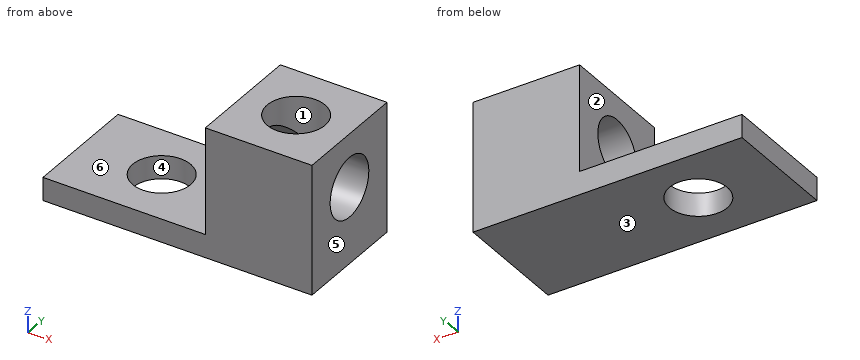
from build123d import *

# Parameters (mm, degrees)
EXTRUDE1_DEPTH      = 12.7
SKETCH2_R           = 3.27152
EXTRUDE2_DEPTH      = 27.071834918
EXTRUDE3_REACH      = 37.096
EXTRUDE3_END_RADIUS = 3.27152
SKETCH3_R           = 3.175
SKETCH4_R           = 3.175
EXTRUDE4_DEPTH      = 35.145763344


with BuildPart() as part:
    # Sketch1 → Extrude1 (new body)
    with BuildSketch(Plane(origin=(0, 0, 0), x_dir=(1, 0, 0), z_dir=(0, 1, 0))):
        Polygon((0, 0), (0, -14.224), (-11.684, -14.224), (-11.684, -2.54), (-29.464, -2.54), (-29.464, 0), align=None)
    extrude(amount=EXTRUDE1_DEPTH)

    # Sketch2 → Extrude2 (cut, through all)
    with BuildSketch(Plane.ZY.offset(11.684)):
        with Locations((8.382, 6.35)):
            Circle(SKETCH2_R)
    extrude(amount=-EXTRUDE2_DEPTH, mode=Mode.SUBTRACT)

    # Extrude3: up to this cylinder (the profile starts outside it)
    extrude3_end = Plane(origin=(-5.842, 6.35, 8.382), z_dir=(-1, 0, 0)) * Cylinder(EXTRUDE3_END_RADIUS, 81.73504, mode=Mode.PRIVATE)
    # Sketch3 → Extrude3 (cut, up to the surface)
    with BuildSketch(Plane.XY.offset(14.224), mode=Mode.PRIVATE) as extrude3_sk1:
        with Locations((-5.842, 6.35)):
            Circle(SKETCH3_R)
    extrude3_tool1 = extrude(extrude3_sk1.sketch, amount=-EXTRUDE3_REACH, mode=Mode.PRIVATE) - extrude3_end
    add(extrude3_tool1.solids().sort_by_distance((-5.842, 6.35, 14.224))[0], mode=Mode.SUBTRACT)

    # Sketch4 → Extrude4 (cut, through all)
    with BuildSketch(Plane.XY.offset(2.54)):
        with Locations((-20.574, 6.35)):
            Circle(SKETCH4_R)
    extrude(amount=-EXTRUDE4_DEPTH, mode=Mode.SUBTRACT)


solid = part.part
CAD build for the part. Positions are in the model's coordinates, mm. Face numbers are marked on the shaded views. A direction names the side the tool comes from. Round coordinates to 2 decimals unless told otherwise and drop trailing zeros. Write each loop counter-clockwise with the first axis right and the second up, starting at its lowest first coordinate (ties: lowest second). Pieces come first, ordered by that corner, then holes. Notation, with made-up numbers: M 79.25,49 L 126.25,49 A18 cw 126.25,54 Z; hole C 86.5,-17.5 d3. An arc over 180 degrees is marked long. Use a Markdown table: item, result. Add a question column.
1. Flat gauge pins, fed straight in: P1, Ø4, axis at x = -24.5, y = 4, coming from the +Z side; P2, Ø3.5, axis at y = 3.5, z = 8, coming from the -X side; P3, Ø4, axis at x = -5.842, y = 6.35, coming from the +Z side; P4, Ø5, axis at x = -20.574, y = 6.35, coming from the +Z side. Where does each tip first touch, or does it go through?
2. Slice it at C-C on y = 1. Give the cut face in (x, z), then the cut area to 3 significant figures.
3. 3-axis set-ups, long thin cutter, end or side, ignore diameter. For the marked faces 1, 2 and 3: which of +Z, -Z, +X, -X, +Y, -Y reach the whole face in a straight line?
4. Pull direction X, two halves, no side cores. Call the marked faces 4, 5 and 6: released by +X, released by -X, zero draft, split by the parting line, or undercut.
5. Drill centre lines: probe 1 along X at (y, z) = (6.35, 12.55); probe 2 along X at (y, z) = (1, 12); probe 3 along Y at (x, z) = (-6.25, 8.25). Where is each one in solid material? Low to high.
6. Slice it at B-B on z = 10.25. Give the cut face in (x, y) (3 decimals).
7. Slice it at A-A on y = 6.35. Give the cut face in (x, z), then the cut area to 3 significant figures.
8. Slice it at D-D on x = -10.25. Give the cut face in (y, z), then the cut area to 3 significant figures.
Reply:
| question | item | result |
|---|---|---|
| 1 | P1 | stops at z = 2.54 |
| 1 | P2 | stops at x = -11.68 |
| 1 | P3 | stops at z = 5.79 |
| 1 | P4 | passes through |
| 2 | outline | M -29.46,0 L 0,0 L 0,14.22 L -11.68,14.22 L -11.68,2.54 L -29.46,2.54 Z |
| 2 | area | 211 mm^2 |
| 3 | face 1 | +Z |
| 3 | face 2 | +Z, -X, +Y, -Y |
| 3 | face 3 | -Z, +X, -X, +Y, -Y |
| 4 | face 4 | undercut |
| 4 | face 5 | released by +X |
| 4 | face 6 | zero draft |
| 5 | probe 1 | x = -11.68 to -9.02, -2.67 to 0 |
| 5 | probe 2 | x = -11.68 to 0 |
| 5 | probe 3 | y = 0 to 3.08, 9.62 to 12.7 |
| 6 | outline | M -11.684,0 L 0,0 L 0,3.664 L -4.149,3.664 A3.175 cw -7.535,3.664 L -11.684,3.664 Z; M -11.684,9.036 L -7.535,9.036 A3.175 cw -4.149,9.036 L 0,9.036 L 0,12.7 L -11.684,12.7 Z |
| 7 | outline | M -29.46,0 L -23.75,0 L -23.75,2.54 L -29.46,2.54 Z; M -17.4,0 L 0,0 L 0,5.11 L -11.68,5.11 L -11.68,2.54 L -17.4,2.54 Z; M -11.68,11.65 L -9.02,11.65 L -9.02,14.22 L -11.68,14.22 Z; M -2.67,11.65 L 0,11.65 L 0,14.22 L -2.67,14.22 Z |
| 7 | area | 102 mm^2 |
| 8 | outline | M 0,0 L 12.7,0 L 12.7,14.22 L 0,14.22 Z; hole C 6.35,8.38 d6.54 |
| 8 | area | 147 mm^2 |
